Verification items for the finished model (mm, model axes). A direction names the side the tool comes from. Coordinates: 2 decimals unless noted, no trailing zeros. Write each loop counter-clockwise with the first axis right and the second up, starting at its lowest first coordinate (ties: lowest second). Pieces come first, ordered by that corner, then holes. Notation, with made-up numbers: M 3,-10 L 21,-10 A25 ccw 21,8 Z; hole C -29.75,5.25 d11. An arc over 180 degrees is marked long. One line per item, written item: value.
Autodesk Inventor part; units mm, degrees
ref_plane "YZ Plane" through (0, 0, 0) normal (1, 0, 0) x (0, 1, 0)
ref_plane "XZ Plane" through (0, 0, 0) normal (0, 1, 0) x (-1, 0, 0)
ref_plane "XY Plane" through (0, 0, 0) normal (0, 0, 1) x (1, 0, 0)
sketch "Sketch1" plane through (0, 0, 0) normal (0, 0, 1) x (1, 0, 0)
  point P0 (0, 0)
sketch "Sketch2" plane through (0, 0, 0) normal (0, 0, 1) x (1, 0, 0)
  line L0 (-270, 130) -> (30, 130)
  line L1 (30, 130) -> (30, 107)
  line L2 (30, 107) -> (-270, 107)
  line L3 (-270, 107) -> (-270, 130)
  line L4 (0, 0) -> (80, 0)
  line L5 (80, 0) -> (80, 150)
  line L6 (80, 150) -> (0, 150)
  line L7 (0, 150) -> (0, 0)
  dimension "d0" = 300
  dimension "d1" = 23
  dimension "d2" = 80
  dimension "d3" = 150
  dimension "d4" = 30
  dimension "d5" = 20
extrude "Extrusion1" add sketch "Sketch2" along normal mid plane 5 contours L0 L7 L2 L3 | L0 L1 L2 L7
sketch "Sketch3" plane through (0, 0, 2.5) normal (0, 0, 1) x (1, 0, 0)
  point P0 (0, 0)
sketch "Sketch4" plane through (0, 0, 2.5) normal (0, 0, 1) x (1, 0, 0)
  point P0 (0, 0)
sketch "Sketch5" plane through (0, 0, -2.5) normal (0, 0, -1) x (-1, 0, 0)
  line L0 (0, 0) -> (-80, 0)
  line L1 (-80, 0) -> (-80, 150)
  line L2 (-80, 150) -> (0, 150)
  line L3 (0, 150) -> (0, 0)
  dimension "d8" = 80
  dimension "d9" = 150
extrude "Extrusion2" add sketch "Sketch5" along normal mid plane 60
sketch "Sketch6" plane through (0, 0, 2.5) normal (0, 0, 1) x (1, 0, 0)
  line L0 (-270, 107) -> (-270, 130)
  line L1 (-270, 130) -> (-230, 130)
  line L2 (-230, 130) -> (-230, 107)
  line L3 (-230, 107) -> (-270, 107)
  line L4 (-270, 107) -> (-270, 130)
  point P0 (0, 0)
  dimension "d12" = 40
  dimension "d13" = 23
extrude "Extrusion3" add sketch "Sketch6" along normal blind 1
sketch "Sketch7" plane through (0, 0, 2.5) normal (0, 0, 1) x (1, 0, 0)
  line L0 (-230.0222, 129.8127) -> (-190.0222, 129.8127)
  line L1 (-190.0222, 129.8127) -> (-190.0222, 106.8127)
  line L2 (-190.0222, 106.8127) -> (-230.0222, 106.8127)
  line L3 (-230.0222, 106.8127) -> (-230.0222, 129.8127)
  point P0 (0, 0)
  dimension "d16" = 40
  dimension "d17" = 23
sketch "Sketch8" plane through (0, 0, 2.5) normal (0, 0, 1) x (1, 0, 0)
  line L0 (-230, 107) -> (-230, 130)
  line L1 (-230, 130) -> (-190, 130)
  line L2 (-190, 130) -> (-190, 107)
  line L3 (-190, 107) -> (-230, 107)
  line L4 (-230, 107) -> (-230, 130)
  line L5 (-190, 130) -> (-150, 130)
  line L6 (-150, 130) -> (-150, 107)
  line L7 (-150, 107) -> (-190, 107)
  line L8 (-190, 107) -> (-190, 130)
  point P0 (0, 0)
  dimension "d18" = 40
  dimension "d19" = 23
  dimension "d20" = 40
  dimension "d21" = 23
extrude "Extrusion4" add sketch "Sketch8" along normal blind 1 contours L2 L5 L6 L7
sketch "Sketch9" plane through (0, 0, 2.5) normal (0, 0, 1) x (1, 0, 0)
  line L0 (-150, 130) -> (-110, 130)
  line L1 (-110, 130) -> (-110, 107)
  line L2 (-110, 107) -> (-150, 107)
  line L3 (-150, 107) -> (-150, 130)
  line L4 (-110, 130) -> (-70, 130)
  line L5 (-70, 130) -> (-70, 107)
  line L6 (-70, 107) -> (-110, 107)
  line L7 (-110, 107) -> (-110, 130)
  point P0 (0, 0)
  dimension "d24" = 40
  dimension "d25" = 23
  dimension "d26" = 40
  dimension "d27" = 23
extrude "Extrusion5" add sketch "Sketch9" along normal blind 1 contours L4 L5 L6 L1
sketch "Sketch10" plane through (0, 0, 2.5) normal (0, 0, 1) x (1, 0, 0)
  line L0 (-70, 130) -> (-70, 107)
  line L1 (-70, 130) -> (-30, 130)
  line L2 (-30, 130) -> (-30, 107)
  line L3 (-30, 107) -> (-70, 107)
  line L4 (-70, 107) -> (-70, 130)
  line L5 (0, 107) -> (0, 130)
  line L6 (-30, 130) -> (0, 130)
  line L7 (0, 130) -> (0, 107)
  line L8 (0, 107) -> (-30, 107)
  line L9 (-30, 107) -> (-30, 130)
  point P0 (0, 0)
  dimension "d30" = 40
  dimension "d31" = 23
  dimension "d32" = 30
  dimension "d33" = 23
extrude "Extrusion6" add sketch "Sketch10" along normal blind 1 contours L6 L5 L8 L2
sketch "Sketch11" plane through (0, 0, 27.5) normal (0, 0, 1) x (1, 0, 0)
  point P0 (0, 0)
sketch "Sketch12" plane through (0, 0, 27.5) normal (0, 0, 1) x (1, 0, 0)
  line L0 (0, 0) -> (80, 0)
  line L1 (80, 0) -> (80, -20)
  line L2 (80, -20) -> (0, -20)
  line L3 (0, -20) -> (0, 0)
  dimension "d36" = 20
extrude "Extrusion7" add sketch "Sketch12" against normal blind 60
properties part number "bar"
Item 1: Scan lines: line 1 (X direction, y = 59.5, z = -8); line 2 (Z direction, x = -220, y = 108). Record each from-to range of solid material in increasing order.
The answers:
line 1: x = 0 to 80
line 2: z = -2.5 to 2.5
Item 2: Cross-section at A-A, the plane y = 28. Enter the section's corners in (x, z).
The answers:
outline: M 0,-32.5 L 80,-32.5 L 80,27.5 L 0,27.5 Z
Item 3: Draft check along X on faces 1 (the face through (-250, 119, 3.5)), 2 (the face through (-210, 119, 2.5)), 3 (the face through (-270, 118, 0)), 4 (the face through (80, 66, -2)). Enter one of: released by +X, released by -X, zero draft, split by the parting line, or undercut.
The answers:
face 1: zero draft
face 2: undercut
face 3: released by -X
face 4: released by +X
Item 4: Cross-section at B-B, the plane x = -44. Enter the section's corners in (y, z).
The answers:
outline: M 107,-2.5 L 130,-2.5 L 130,2.5 L 107,2.5 Z
Item 5: Access from +Z, -Z, +X, -X, +Y, -Y to the whole of each face (thin tool, end or side, straight path). Record for faces 5 (the face through (-90, 119, 3.5)), 6 (the face through (-137, 130, 0)), 7 (the face through (-137, 119, -2.5)).
The answers:
face 5: +Z, -X, +Y, -Y
face 6: +Z, -Z, -X, +Y
face 7: -Z, -X, +Y, -Y
Item 6: Go/stop test with flat-tipped pins: P1, Ø6, axis at x = -73.5, y = 113.5, coming from the -Z side; P2, Ø6.5, axis at x = -116.5, z = 1, coming from the -Y side; P3, Ø18.5, axis at x = -80.5, y = 121, coming from the +Z side. Record where each tip stops, or that it passes through.
The answers:
P1: stops at z = -2.5
P2: stops at y = 107
P3: stops at z = 3.5
